Geometry: see drawing. Coordinates: mm, zero at the bounding-box minimum. A direction names the side the tool comes from. Coordinates: 2 decimals unless noted, no trailing zeros. Order: outer loops, then holes, each group sorted by start corner. A loop starts at its lowest first (then second) coordinate and runs counter-clockwise, first axis right, second up. Notation, with made-up numbers: (78, 39.25) -> (119, 39.25) arc R15 cw to (119, 50.25) -> close; hole circle Ø7 at (62.5, 89). An arc over 180 degrees is marked (long way). Use one line per item in the form item = value.
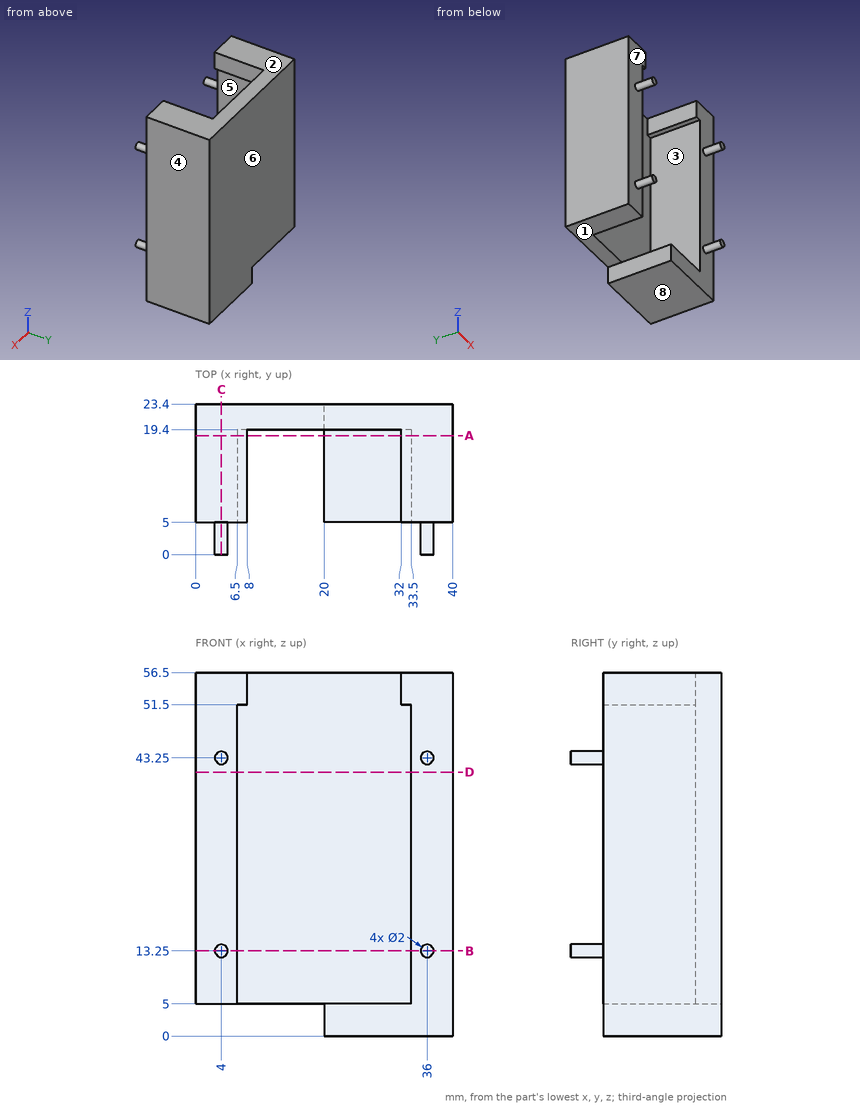
1) Pull-direction query (Z, two-part tool) for the marked faces 6, 7 and 8; classes: released by +Z, released by -Z, zero draft, split by the parting line, or undercut.
Results found:
face_6 = zero draft
face_7 = undercut
face_8 = released by -Z
2) Material intervals for probe 1 along X at (y, z) = (5.25, 45.5); probe 2 along X at (y, z) = (5.75, 54); probe 3 along Y at (x, z) = (38, 3.5), sorted ascending. Write a range as from..to.
Results found:
probe_1 = 0..6.5, 33.5..40
probe_2 = 0..8, 32..40
probe_3 = 5..23.4
3) Access query for the marked faces 1, 2, 3, 4 and 5. Directions: +Z, -Z, +X, -X, +Y, -Y. A direction counts if a zero-diameter tool reaches every point of the face in a straight line with its end or side. Return the directions, or none.
Results found:
face_1 = -Z, -X, +Y, -Y
face_2 = +Z, +X, -X, +Y, -Y
face_3 = -Y
face_4 = +Z, -Z, +X, +Y, -Y
face_5 = -Z, -Y
4) Section D-D, the plane z = 41. Output: boundary loops of the cut face in (x, y), and give its area (3 significant figures).
Results found:
outline = (0, 5) -> (6.5, 5) -> (6.5, 19.4) -> (33.5, 19.4) -> (33.5, 5) -> (40, 5) -> (40, 23.4) -> (0, 23.4) -> close
area = 347 mm2
5) Contact query for flat-ended pins moving along their axis: P1, Ø4, axis at x = 17, z = 42.5, coming from the -Y side; P2, Ø1.5, axis at y = 15, z = 54.5, coming from the -X side; P3, Ø4, axis at x = 24.5, y = 12.5, coming from the +Z side; P4, Ø9, axis at x = 4.5, z = 23.5, coming from the -Y side. Output: stop coordinate, or through.
Results found:
P1 = 19.4
P2 = 0
P3 = 5
P4 = 5
6) Section B-B, the plane z = 13.25. Output: boundary loops of the cut face in (x, y), and give its area (3 significant figures).
Results found:
outline = (0, 5) -> (3, 5) -> (3, 0) -> (5, 0) -> (5, 5) -> (6.5, 5) -> (6.5, 19.4) -> (33.5, 19.4) -> (33.5, 5) -> (35, 5) -> (35, 0) -> (37, 0) -> (37, 5) -> (40, 5) -> (40, 23.4) -> (0, 23.4) -> close
area = 367 mm2
7) Section C-C, the plane x = 4. Output: boundary loops of the cut face in (y, z), and give its area (3 significant figures).
Results found:
outline = (0, 12.25) -> (5, 12.25) -> (5, 5) -> (23.4, 5) -> (23.4, 56.5) -> (5, 56.5) -> (5, 44.25) -> (0, 44.25) -> (0, 42.25) -> (5, 42.25) -> (5, 14.25) -> (0, 14.25) -> close
area = 968 mm2
8) Section A-A, the plane y = 18.5. Output: boundary loops of the cut face in (x, z).
Results found:
outline = (0, 5) -> (6.5, 5) -> (6.5, 51.5) -> (8, 51.5) -> (8, 56.5) -> (0, 56.5) -> close; (20, 0) -> (40, 0) -> (40, 56.5) -> (32, 56.5) -> (32, 51.5) -> (33.5, 51.5) -> (33.5, 5) -> (20, 5) -> close
